Input: part model. Units: mm. Frame: model coordinates. Face numbers are marked on the shaded views. A direction names the side the tool comes from. Coordinates: 2 decimals unless noted, no trailing zeros. Loops run counter-clockwise (first coordinate to the right, second up) from the corner with the lowest first, then second, coordinate; pieces in that order, holes last.
Item 1: Section D-D on x = 72. Return loops of the section in (y, z), and give its area (3 significant figures).
Item 2: Ray query, line 1 along Y through (x, z) = (6, 14); line 2 along X through (y, z) = (3.5, 11.5); line 3 along Z through (x, y) = (73, 38.5). Return the intervals inside material, ascending.
Item 3: Reachability of the marked faces 1, 2 and 3 from +Z, -Z, +X, -X, +Y, -Y: full face, straight path, thin tool, end or side. Return the list, or none.
Item 4: Section C-C on z = 5. Return loops of the section in (x, y), and give its area (3 significant figures).
Item 5: Section B-B on x = 33. Return loops of the section in (y, z).
Item 6: Section A-A on y = 24. Return loops of the section in (x, z).
Item 7: Contact query for a flat-ended pin moving along its axis: P1, Ø4, axis at y = 35, z = 11.5, coming from the +X side. Output: stop coordinate, or through.
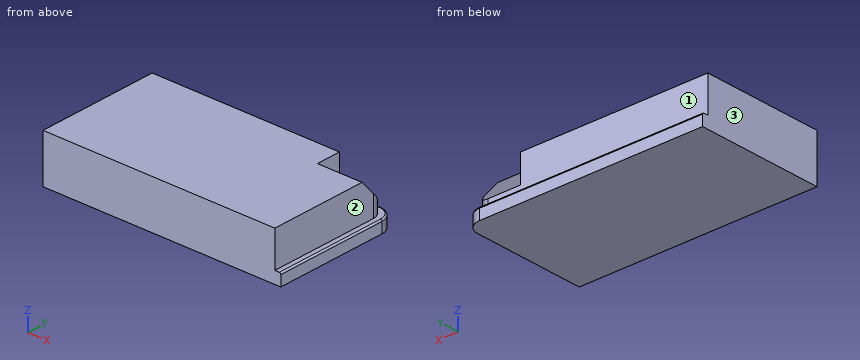
```python
from build123d import *

# Parameters (mm, degrees)
F0_W     = 80
F0_H     = 43
F1_DEPTH = 4
F2_W     = 78
F2_H     = 41
F3_DEPTH = 12
F4_R     = 5
F5_R     = 0.5
F7_DEPTH = 15
F8_R     = 4


# Not quite as in the source:
# - a feature of the source that left no trace in its solid (it failed there, or was rolled back) is left out


with BuildPart() as f1:
    # F0 (on Top) → F1 (new body)
    with BuildSketch(Plane.XY):
        with Locations((40, 21.5)):
            Rectangle(F0_W, F0_H)
    extrude(amount=F1_DEPTH)

    # F2 (on face) → F3 (join)
    with BuildSketch(Plane.XY.offset(4)):
        with Locations((39, 20.5)):
            Rectangle(F2_W, F2_H)
    extrude(amount=F3_DEPTH)

    # F4
    f4_edges = [f1.edges().sort_by_distance(p)[0] for p in [
        (80, 43, 2),
    ]]
    fillet(f4_edges, radius=F4_R)

    # F5
    f5_edges = [f1.edges().sort_by_distance(p)[0] for p in [
        (37.5, 43, 4),
        (78.535534, 41.535534, 4),
        (80, 19, 4),
    ]]
    fillet(f5_edges, radius=F5_R)

    # F6 (on face) → F7 (cut)
    with BuildSketch(Plane.YZ.offset(78)):
        Polygon((41, 16), (32.7275320888, 16), (41, 6.6185845062), align=None)
    extrude(amount=-F7_DEPTH, mode=Mode.SUBTRACT)

    # F8
    f8_edges = [f1.edges().sort_by_distance(p)[0] for p in [
        (78, 41, 5.309292),
    ]]
    fillet(f8_edges, radius=F8_R)


solid = f1.part
```
Results found:
1. outline: (0, 0) - (43, 0) - (43, 3.5) arc R0.5 ccw to (42.5, 4) - (41, 4) - (41, 6.62) - (32.73, 16) - (0, 16) - close
1. area: 625 mm2
2. line 1: y = 0 to 41
2. line 2: x = 0 to 78
2. line 3: z = 0 to 9.45
3. face 1: +Z, +X, -X, +Y
3. face 2: +Z, +X, +Y, -Y
3. face 3: +Z, -Z, -X, +Y, -Y
4. outline: (0, 0) - (78, 0) - (78, 37) arc R4 ccw to (74, 41) - (0, 41) - close
4. area: 3,190 mm2
5. outline: (0, 0) - (43, 0) - (43, 3.5) arc R0.5 ccw to (42.5, 4) - (41, 4) - (41, 16) - (0, 16) - close
6. outline: (0, 0) - (80, 0) - (80, 3.5) arc R0.5 ccw to (79.5, 4) - (78, 4) - (78, 16) - (0, 16) - close
7. P1: stops at x = 78
